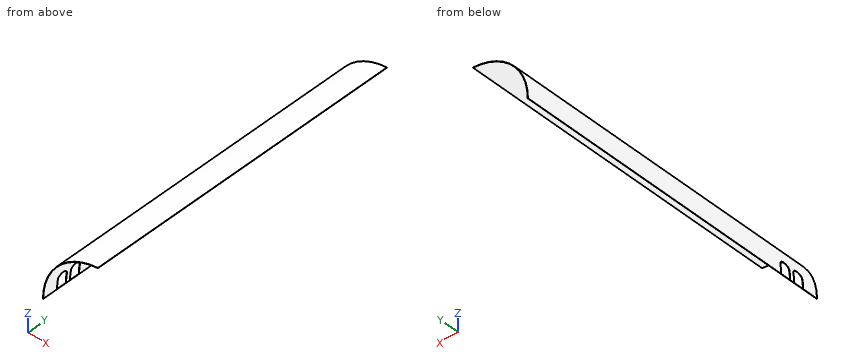
Autodesk Inventor part; units mm, degrees
ref_plane "Work Plane1" through (-303.1515, 0, 50.567) normal (-0.9863719, 0, 0.1645312) x (0, -1, 0)
ref_plane "YZ Plane" through (0, 0, 0) normal (1, 0, 0) x (0, 1, 0)
ref_plane "XZ Plane" through (0, 0, 0) normal (0, 1, 0) x (-1, 0, 0)
sketch "Sketch1" plane through (0, 0, 0) normal (0, 1, 0) x (-1, 0, 0)
  arc A0 (307.34, 0) -> (25.3968, 306.2889) centre (0, 0) ccw
  line L0 (0, 0) -> (25.3968, 306.2889) construction
  line L1 (0, 0) -> (307.34, 0) construction
  arc A1 (306.07, 0) -> (25.2919, 305.0232) centre (0, 0) ccw
  line L2 (0, 0) -> (25.2919, 305.0232) construction
  line L3 (0, 0) -> (306.07, 0) construction
  line L4 (306.07, 0) -> (307.34, 0)
  line L5 (25.2919, 305.0232) -> (25.3968, 306.2889)
  dimension "d0" = 307.34
  dimension "d1" = 85.26
  dimension "d2" = 306.07
  dimension "d3" = 85.26
extrude "Extrusion1" add sketch "Sketch1" along normal blind 1625.6
sketch "Sketch2" plane through (0, 0, 0) normal (0, 1, 0) x (-1, 0, 0)
  arc A0 (307.34, 0) -> (303.1515, 50.567) centre (0, 0) ccw
  line L0 (0, 0) -> (303.1515, 50.567) construction
  line L1 (0, 0) -> (307.34, 0) construction
  arc A1 (307.34, 0) -> (290.6829, 99.8065) centre (0, 0) ccw
  line L2 (0, 0) -> (290.6829, 99.8065) construction
  line L3 (0, 0) -> (307.34, 0) construction
  arc A2 (123.4855, 281.4413) -> (25.3968, 306.2889) centre (0, 0) ccw
  line L4 (0, 0) -> (123.4855, 281.4413) construction
  line L5 (0, 0) -> (25.3968, 306.2889) construction
  dimension "d6" = 307.34
  dimension "d7" = 9.47
  dimension "d14" = 18.95
  dimension "d15" = 18.95
ref_plane "Work Plane1" through (-303.1515, 0, 50.567) normal (-0.9863719, 0, 0.1645312) x (0, -1, 0)
sketch "Sketch3" plane through (-303.1515, 0, 50.567) normal (-0.9863719, 0, 0.1645312) x (0, -1, 0)
  circle A0 centre (-103.1875, 0) radius 25.4
  line L0 (0, 297.9362) -> (0, -50.567)
  line L1 (0, -50.3581) -> (-1625.6, -50.3581)
  line L2 (-128.5875, 0) -> (-77.7875, 0)
  line L3 (-77.7875, 0) -> (-77.7875, -50.3581)
  line L4 (-77.7875, -50.3581) -> (-128.5875, -50.3581)
  line L5 (-128.5875, -50.3581) -> (-128.5875, 0)
  circle A1 centre (-176.2125, 0) radius 25.4
  line L6 (-201.6125, 0) -> (-150.8125, 0)
  line L7 (-150.8125, 0) -> (-150.8125, -50.3581)
  line L8 (-150.8125, -50.3581) -> (-201.6125, -50.3581)
  line L9 (-201.6125, -50.3581) -> (-201.6125, 0)
  point P0 (0, 0)
  dimension "d8" = 50.8
  dimension "d10" = 50.8
  dimension "d9" = 103.1875
  dimension "d11" = 176.2125
extrude "Extrusion2" cut sketch "Sketch3" against normal blind 25.4
properties part number "EDM Middle Shield Part 4"
Build history of the part. All positions in model axes, mm. Round coordinates to 2 decimals unless told otherwise and drop trailing zeros. Write each loop counter-clockwise with the first axis right and the second up, starting at its lowest first coordinate (ties: lowest second). Pieces come first, ordered by that corner, then holes.
1) Band-saw the part on C-C, the plane x = -82. List the corners of the cut face in (y, z).
2) Drill centre lines: probe 1 along X at (y, z) = (1483.5, 92.5); probe 2 along X at (y, z) = (427, 74.5); probe 3 along Z at (x, y) = (-175.5, 881). Where is each one in solid material? Low to high.
3) Pin check, flat tips, straight feed: pin 1 (8 mm diameter, centred on y = 228, z = 243.5, fed in from +X); pin 2 (2.5 mm diameter, centred on x = -304, z = 16.5, fed in from -Y); pin 3 (10 mm diameter, centred on x = -157.5, y = 501, fed in from -Z); pin 4 (4 mm diameter, centred on x = -90.5, y = 1174, fed in from -Z). Stop position of each tip, or through.
4) Band-saw the part on B-B, the plane y = 1422. List the corners of the cut face in (x, z), and give its area (3 significant figures).
Ans:
1. outline: (0, 294.88) - (1625.6, 294.88) - (1625.6, 296.2) - (0, 296.2) - close
2. probe 1: x = -293.09 to -291.76
2. probe 2: x = -298.17 to -296.86
2. probe 3: z = 250.76 to 252.3
3. pin 1: stops at x = -180.06
3. pin 2: passes through
3. pin 3: stops at z = 259.37
3. pin 4: stops at z = 291.76
4. outline: (-307.34, 0) - (-306.07, 0) arc R306.07 cw to (-25.29, 305.02) - (-25.4, 306.29) arc R307.34 ccw to start
4. area: 580 mm2
